Check sheet for the modelled part. Datum: model origin and axes. Units: mm. Give positions to 0.01 mm unless a question says otherwise; leave off trailing zeros. Use CSV: the item, a comma, the result in double quotes.
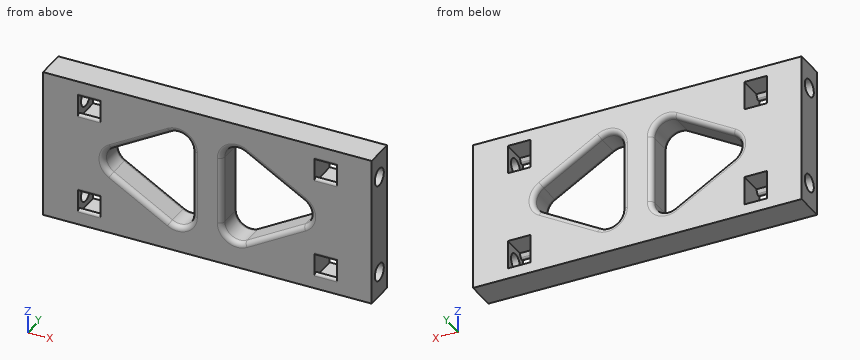
from build123d import *

# Parameters (mm, degrees)
SKETCH1_W           = 30
SKETCH1_H           = 6
BOSS_EXTRUDE1_DEPTH = 33
SKETCH2_R           = 1.75
CUT_EXTRUDE1_DEPTH  = 7
CUT_EXTRUDE2_DEPTH  = 4.5
CUT_EXTRUDE3_DEPTH  = 7
FILLET1_R           = 3
FILLET2_R           = 1
FILLET3_R           = 0.5


with BuildPart() as part:
    # Sketch1 → Boss-Extrude1 (new body, symmetric)
    with BuildSketch(Plane(origin=(0, 0, 0), x_dir=(0, 0, -1), z_dir=(1, 0, 0))):
        Rectangle(SKETCH1_W, SKETCH1_H)
    extrude(amount=BOSS_EXTRUDE1_DEPTH, both=True)

    # Sketch2 → Cut-Extrude1 (cut)
    with BuildSketch(Plane(origin=(33, 0, 0), x_dir=(0, 0, -1), z_dir=(1, 0, 0))):
        with Locations((-10, 0)):
            Circle(SKETCH2_R)
        with Locations((10, 0)):
            Circle(SKETCH2_R)
    cut_extrude1 = extrude(amount=-CUT_EXTRUDE1_DEPTH, mode=Mode.SUBTRACT)

    # Sketch3 → Cut-Extrude2 (cut)
    with BuildSketch(Plane(origin=(26, 0, 0), x_dir=(0, 0, -1), z_dir=(1, 0, 0))):
        Polygon((-12.875, 3), (-12.875, 1.659882024), (-10.553847577, 3), align=None)
        Polygon((-10.553847577, 3), (-12.875, 1.659882024), (-12.875, -1.659882024), (-10, -3.319764048), (-7.125, -1.659882024), (-7.125, 1.659882024), (-9.446152423, 3), align=None)
        Polygon((-10, 3.319764048), (-10.553847577, 3), (-9.446152423, 3), align=None)
        Polygon((-7.125, 3), (-9.446152423, 3), (-7.125, 1.659882024), align=None)
        Polygon((12.875, 3), (7.125, 3), (7.125, 1.659882024), (7.125, -1.659882024), (10, -3.319764048), (12.875, -1.659882024), (12.875, 1.659882024), align=None)
    cut_extrude2 = extrude(amount=-CUT_EXTRUDE2_DEPTH, mode=Mode.SUBTRACT)

    # Mirror1: Cut-Extrude1, Cut-Extrude2 across plane
    add(cut_extrude1.mirror(Plane(origin=(0, 0, 0), x_dir=(0, 0, 1), z_dir=(1, 0, 0))), mode=Mode.SUBTRACT)
    add(cut_extrude2.mirror(Plane(origin=(0, 0, 0), x_dir=(0, 0, 1), z_dir=(1, 0, 0))), mode=Mode.SUBTRACT)

    # Sketch4 → Cut-Extrude3 (cut, through all)
    with BuildSketch(Plane(origin=(0, 3, 0), x_dir=(1, 0, 0), z_dir=(0, 1, 0))):
        Polygon((-3, -12), (-3, 12), (-23.75, 0), align=None)
        Polygon((23.75, 0), (3, 12), (3, -12), align=None)
    extrude(amount=-CUT_EXTRUDE3_DEPTH, mode=Mode.SUBTRACT)

    # Fillet1
    fillet1_edges = [part.edges().sort_by_distance(p)[0] for p in [
        (-23.75, 0, 0),
        (-3, 0, -12),
        (-3, 0, 12),
        (23.75, 0, 0),
        (3, 0, 12),
        (3, 0, -12),
    ]]
    fillet(fillet1_edges, radius=FILLET1_R)

    # Fillet2
    fillet2_edges = [part.edges().sort_by_distance(p)[0] for p in [
        (13.380621084, 3, -5.996749253),
        (13.380621084, -3, -5.996749253),
        (13.380621084, 3, 5.996749253),
        (13.380621084, -3, 5.996749253),
        (3, 3, 0),
        (3, -3, 0),
        (-3, 3, 0),
        (-3, -3, 0),
        (-13.380621084, 3, 5.996749253),
        (-13.380621084, -3, 5.996749253),
        (-13.380621084, 3, -5.996749253),
        (-13.380621084, -3, -5.996749253),
        (20.757491656, 3, 0),
        (20.757491656, -3, 0),
        (4.500937921, 3, 9.398130742),
        (4.500937921, -3, 9.398130742),
        (4.500937921, 3, -9.398130742),
        (4.500937921, -3, -9.398130742),
        (-4.500937921, 3, 9.398130742),
        (-4.500937921, -3, 9.398130742),
        (-20.757491656, 3, 0),
        (-20.757491656, -3, 0),
        (-4.500937921, 3, -9.398130742),
        (-4.500937921, -3, -9.398130742),
    ]]
    fillet(fillet2_edges, radius=FILLET2_R)

    # Fillet3
    fillet3_edges = [part.edges().sort_by_distance(p)[0] for p in [
        (23.75, -3, 10.553847577),
        (23.75, -3, 9.446152423),
        (23.75, -3, -9.446152423),
        (23.75, -3, -10.553847577),
        (-23.75, -3, 9.446152423),
        (-23.75, -3, 10.553847577),
        (-23.75, -3, -10.553847577),
        (-23.75, -3, -9.446152423),
    ]]
    fillet(fillet3_edges, radius=FILLET3_R)


solid = part.part
1. Scan lines: line 1 along Z through (x, y) = (23.5, 1.5) (3 decimals); line 2 along Y through (x, z) = (28.5, 10); line 3 along X through (y, z) = (1, 0.5). Record each from-to range of solid material in increasing order.
Completed:
line 1,"z = -15 to -12.875, -7.125 to 7.125, 12.875 to 15"
line 2,"y = -3 to -1.75, 1.75 to 3"
line 3,"x = -33 to -20.72, -3 to 3, 20.72 to 33"
2. Go/stop test with flat-tipped pins: pin 1 Ø3 at (y, z) = (1, -10.5) entering from -X; pin 2 Ø3 at (y, z) = (0, -10) entering from +X. Record where each tip stops, or that it passes through.
Completed:
pin 1,"stops at x = -33"
pin 2,"stops at x = 21.5"
3. Sectioned sample at A-A, the plane z = -2. State how many separate pieces and enclosed holes the cut face has, and give its area (3 significant figures).
Completed:
separate pieces,"3"
enclosed holes,"0"
area,"190 mm²"
